Autodesk Inventor part; units mm, degrees
ref_plane "YZ Plane" through (0, 0, 0) normal (1, 0, 0) x (0, 1, 0)
ref_plane "XZ Plane" through (0, 0, 0) normal (0, 1, 0) x (-1, 0, 0)
ref_plane "XY Plane" through (0, 0, 0) normal (0, 0, 1) x (1, 0, 0)
sketch "Sketch1" plane through (59.7334, 64.5979, 5.1545) normal (1, 0, 0) x (0, 1, 0)
  line L0 (18.8189, 17.1759) -> (22.8279, 17.1759)
  line L1 (18.8189, -4.3241) -> (22.8279, -4.3241)
  line L2 (22.3279, -4.8241) -> (19.3338, -4.8241)
  arc A0 (-48.3948, 28.867) -> (-62.6447, 12.9256) centre (-53.5949, 19.1757) ccw
  line L3 (-48.3948, 28.867) -> (-28.1429, 18.0072)
  line L4 (-24.8341, 17.1759) -> (22.8279, 17.1759)
  line L5 (22.8279, 17.1759) -> (22.8279, -4.3241)
  line L6 (22.8279, -4.3241) -> (22.8279, -4.8241)
  line L7 (22.8279, -4.8241) -> (22.3279, -4.8241)
  line L8 (22.3279, -4.8241) -> (-50.3885, -4.8241)
  line L9 (-50.3885, -4.8241) -> (-62.6447, 12.9256)
  arc A1 (-28.1429, 18.0072) -> (-24.8341, 17.1759) centre (-24.8333, 24.1792) ccw
  point P0 (-48.3934, 28.8694)
  point P1 (0.4728, 17.1759)
  point P2 (-13.5862, 6.178)
sketch "Sketch2" plane through (47.0121, 65.2772, 22.3304) normal (0, 0, 1) x (1, 0, 0)
  line L0 (17.0615, 5.4672) -> (24.4547, 9.7356)
  line L1 (24.4547, 9.7356) -> (24.4547, 16.9356)
  line L2 (24.4547, 16.9356) -> (22.0224, 21.1485)
  arc A0 (22.0224, 21.1485) -> (19.2903, 21.8806) centre (20.2903, 20.1485) ccw
  line L3 (22.0224, 21.1485) -> (20.2903, 20.1485) construction
  line L4 (19.2903, 21.8806) -> (20.2903, 20.1485) construction
  line L5 (19.2903, 21.8806) -> (4.2935, 13.2221)
  arc A1 (4.2935, 13.2221) -> (3.3088, 11.2431) centre (5.2935, 11.4901) ccw
  arc A2 (-25.8662, 11.2431) -> (3.3088, 11.2431) centre (-11.2787, 9.4277) ccw
  arc A3 (-25.8662, 11.2431) -> (-26.8509, 13.2221) centre (-27.8509, 11.4901) ccw
  line L6 (-26.8509, 13.2221) -> (-41.8477, 21.8806)
  arc A4 (-41.8477, 21.8806) -> (-44.5798, 21.1485) centre (-42.8477, 20.1485) ccw
  line L7 (-44.5798, 21.1485) -> (-47.0121, 16.9356)
  line L8 (-47.0121, 16.9356) -> (-47.0121, 16.9356)
  line L9 (-47.0121, 9.7356) -> (-39.9003, 5.6296)
  line L10 (-39.926, 5.6445) -> (-39.2899, 5.1683)
  line L11 (-39.926, 5.6445) -> (-47.0121, 9.7356)
  arc A5 (-28.8787, -13.5153) -> (-39.926, 5.6445) centre (-55.4557, -16.0746) ccw
  line L12 (12.7213, -0.2066) -> (17.0615, 5.4672)
  line L13 (12.7213, -65.2726) -> (12.7213, -49.0741)
  line L14 (12.7213, -65.2726) -> (12.7213, -25.5127)
  line L15 (12.7213, -65.2726) -> (-28.8787, -65.2726)
  line L16 (12.7213, -25.5127) -> (12.7213, -0.2066)
  line L17 (-28.8787, -65.2726) -> (-28.8787, -13.5153)
  line L18 (-47.0121, 9.7356) -> (-47.0121, 16.9356)
  line L19 (-6.7787, -27.2723) -> (-15.7787, -27.2723)
  line L20 (-6.7787, -27.2723) -> (-15.7787, -27.2723)
  line L21 (-6.7787, -27.2723) -> (-15.7787, -27.2723)
  line L22 (-15.7787, -27.2723) -> (-15.7787, -3.6713)
  line L23 (-15.7787, -3.6713) -> (-6.7787, -3.6713)
  line L24 (-6.7787, -3.6713) -> (-6.7787, -27.2723)
  arc A6 (-15.7787, -6.4085) -> (-17.3582, -3.9562) centre (-18.4721, -6.4085) ccw
  arc A7 (-5.218, -3.9648) -> (-6.7787, -6.384) centre (-4.1232, -6.384) ccw
  point P0 (-47.0121, -65.2772)
  point P1 (12.7213, -49.0728)
  point P2 (12.7213, -63.3241)
  point P3 (-15.7787, -5.7822)
  dimension "d3" = 2
  dimension "d4" = 90
  dimension "d5" = 2
  dimension "d6" = 26.7
  dimension "d7" = 2
  dimension "d8" = 90
  dimension "d13" = 0
extrude "Extrusion1" add sketch "Sketch1" along normal mid plane 200
extrude "Extrusion2" cut sketch "Sketch2" along normal mid plane 200 contours L12 L16 L14 L13 L15 L17 A5 L9 L18 L7 A4 L6 A3 A2 A6 L22 L19 L24 A7 A1 L5 A0 L2 L1 L0 keep common part
sketch "Sketch5" plane through (35.7334, 74.705, 22.3304) normal (0, 0, 1) x (1, 0, 0)
  point P0 (-35.7334, -74.705)
sketch "Sketch3" plane through (66.3024, 87.1578, 22.3304) normal (-0.4999998, 0.8660255, 0) x (0.8660255, 0.4999998, 0)
  ellipse E0 centre (-8.9999, 10.9997) end of major axis (-4.913, 11.323) minor radius 4.0997
  point P0 (-100.9985, 22.3304)
sketch "Sketch4" plane through (20.1613, 78.4993, 22.3304) normal (0.5000005, 0.8660251, 0) x (0.8660251, -0.5000005, 0)
  ellipse E0 centre (-8.3172, 10.9997) end of major axis (-5.344, 8.1771) minor radius 4.0996
  point P0 (21.7896, 22.3304)
sketch "Sketch6" plane through (18.1334, 14.2094, 0.3304) normal (-1, 0, 0) x (0, 0, 1)
  point P0 (-0.3304, -14.2094)
hole "Hole1" at (58.5083, 82.6578, 11.3306) direction (0.4999998, -0.8660255, 0) diameter 8 end through all
hole "Hole2" at (12.9584, 82.6579, 11.3307) direction (-0.5000005, -0.8660251, 0) diameter 8 end through all
hole "Hole3" at (59.7334, 51.0116, 11.3325) at (59.7334, 11.003, 24.3302) direction (-1, 0, 0) diameter 8 end through all
properties part number "YZ_Roller"
Here's how the part is built. I have some questions about the finished solid (model axes, mm). A direction names the side the tool comes from. Coordinates: 2 decimals unless noted, no trailing zeros. Order: outer loops, then holes, each group sorted by start corner. A loop starts at its lowest first (then second) coordinate and runs counter-clockwise, first axis right, second up.
Item 1: If we mould it in two halves opening along Z, with no side actions, what happens to faces 4 (the face through (38.64, 37.71, 22.64)), 5 (the face through (1.233, 84.349, 11.176)), 6 (the face through (38.642, 9.802, 20.515)), 7 (the face through (38.64, 2.67, 31.51))? For each: +Z half, -Z half, draft (parallel to the pull), parting line (faces both ways), or undercut.
Result sheet:
face 4: +Z half
face 5: draft
face 6: undercut
face 7: parting line
Item 2: For P1, Ø9.5, axis at x = 21, y = 55.5, coming from the +Z side; P2, Ø10.5, axis at y = 48.5, z = 11, coming from the +X side; P3, Ø6, axis at x = 17.5, z = 20.5, coming from the -Y side; P4, Ø5, axis at y = 51.01, z = 11.33, coming from the +X side, each with a flat end and sliding along its axis, tell me the tip position at first contact or that it passes through.
Result sheet:
P1: stops at z = 22.33
P2: stops at x = 59.73
P3: stops at y = 0.04
P4: passes through
Item 3: If we section it at C-C on x = 35.5: List the corners of the cut face in (y, z) for me (1 decimal).
Result sheet:
outline: (2, 18.1) - (14.2, 0.3) - (38, 0.3) - (38, 22.6) arc R7 cw to (36.5, 23.2) - (16.2, 34) arc R11 ccw to start; hole circle Ø8 at (11, 24.3)
Item 4: If we section it at A-A on y = 45.5: List the corners of the cut face in (x, z) for me, plus the area to 3 significant figures.
Result sheet:
outline: (18.13, 0.33) - (31.23, 0.33) - (31.23, 22.33) - (18.13, 22.33) - close; (40.23, 0.33) - (59.73, 0.33) - (59.73, 22.33) - (40.23, 22.33) - close
area: 717 mm2
Item 5: If we section it at D-D on z = 16.5: List the corners of the cut face in (x, y) for me.
Result sheet:
outline: (0, 75.01) - (7.09, 70.92) arc R26.7 cw to (18.13, 51.76) - (18.13, 3.04) - (59.73, 3.04) - (59.73, 65.07) - (64.07, 70.74) - (71.47, 75.01) - (71.47, 82.21) - (69.03, 86.43) arc R2 ccw to (66.3, 87.16) - (51.31, 78.5) arc R2 ccw to (50.32, 76.52) arc R14.7 cw to (41.79, 61.31) arc R2.66 ccw to (40.23, 58.89) - (40.23, 38) - (31.23, 38) - (31.23, 58.87) arc R2.69 ccw to (29.65, 61.32) arc R14.7 cw to (21.15, 76.52) arc R2 ccw to (20.16, 78.5) - (5.16, 87.16) arc R2 ccw to (2.43, 86.43) - (0, 82.21) - close
Item 6: For faces 1 (the face through (36, 38.005, 11)), 2 (the face through (22.97, 67.41, 11.18)), 3 (the face through (18.133, 26, 14)), which set-ups out of +Z, -Z, +X, -X, +Y, -Y let a thin tool reach every point of the face, with its end or its side?
Result sheet:
face 1: +Z, -Z, +Y
face 2: +Z, -Z
face 3: +Z, -Z, -X, -Y
Item 7: I need wall thicknesses on line 1 (X direction, y = 40, z = 4); line 2 (Y direction, x = 58.5, z = 22); line 3 (X direction, y = 14, z = 28). Which ranges of each line are inside material? Lowest first, please.
Result sheet:
line 1: x = 18.13 to 31.23, 40.23 to 59.73
line 2: y = 0.25 to 7.75, 14.25 to 82.65
line 3: x = 18.13 to 59.73
Item 8: If we section it at B-B on x = 23: List the corners of the cut face in (y, z) for me (1 decimal), plus the area to 3 significant figures.
Result sheet:
outline: (2, 18.1) - (14.2, 0.3) - (67.4, 0.3) - (67.4, 22.3) - (39.8, 22.3) arc R7 cw to (36.5, 23.2) - (16.2, 34) arc R11 ccw to start; hole circle Ø8 at (11, 24.3); hole circle Ø8 at (51, 11.3)
area: 1,540 mm2
